CAD build for the part. Positions are in the model's coordinates, mm. Face numbers are marked on the shaded views. A direction names the side the tool comes from. Coordinates: 2 decimals unless noted, no trailing zeros. Write each loop counter-clockwise with the first axis right and the second up, starting at its lowest first coordinate (ties: lowest second). Pieces come first, ordered by that corner, then holes. Notation, with made-up numbers: M 28.25,63.25 L 77.25,63.25 A24 cw 77.25,73.25 Z; hole C -36.5,63.5 d1. An arc over 180 degrees is marked long. Put each result on its own line as item: value. Start each with the question number.
```python
from build123d import *

# Parameters (mm, degrees)
F0_W     = 139.7
F0_H     = 133.35
F1_DEPTH = 38.1
F2_T     = -1.5
F4_DEPTH = 1.5


# Not quite as in the source:
# - a pattern or mirror of a feature is missing from the dataset's text; its kind, count and spacing are read off the source's solid


with BuildPart() as f1:
    # F0 (on Top) → F1 (new body)
    with BuildSketch(Plane.XY):
        Rectangle(F0_W, F0_H)
    extrude(amount=F1_DEPTH)

    # F2
    f2_openings = [f1.faces().sort_by_distance(p)[0] for p in [
        (0, 0, 38.1),
    ]]
    offset(amount=F2_T, openings=f2_openings)

    # F3 (on face) → F4 (cut)
    with BuildSketch(Plane.XZ.offset(66.675)):
        with BuildLine():
            Line((19.05, 20.55), (-19.05, 20.55))
            ThreePointArc((-19.05, 20.55), (0, 1.5), (19.05, 20.55))
        make_face()
        with BuildLine():
            Line((-19.05, 38.1), (-19.05, 20.55))
            ThreePointArc((-19.05, 20.55), (-15.8753360228, 31.0797771184), (-7.4094534211, 38.1))
            Line((-7.4094534211, 38.1), (-19.05, 38.1))
        make_face()
        with BuildLine():
            ThreePointArc((-7.4094534211, 38.1), (-15.8753360228, 31.0797771184), (-19.05, 20.55))
            Line((-19.05, 20.55), (19.05, 20.55))
            ThreePointArc((19.05, 20.55), (15.8753360228, 31.0797771184), (7.4094534211, 38.1))
            Line((7.4094534211, 38.1), (-7.4094534211, 38.1))
        make_face()
        with BuildLine():
            ThreePointArc((7.4094534211, 38.1), (15.8753360228, 31.0797771184), (19.05, 20.55))
            Line((19.05, 20.55), (19.05, 38.1))
            Line((19.05, 38.1), (7.4094534211, 38.1))
        make_face()
        with BuildLine():
            ThreePointArc((7.4094534211, 38.1), (0, 39.6), (-7.4094534211, 38.1))
            Line((-7.4094534211, 38.1), (7.4094534211, 38.1))
        make_face()
    f4 = extrude(amount=-F4_DEPTH, mode=Mode.SUBTRACT)

    # F4_copies: F4 across plane
    add(f4.mirror(Plane.ZX), mode=Mode.SUBTRACT)


solid = f1.part
```
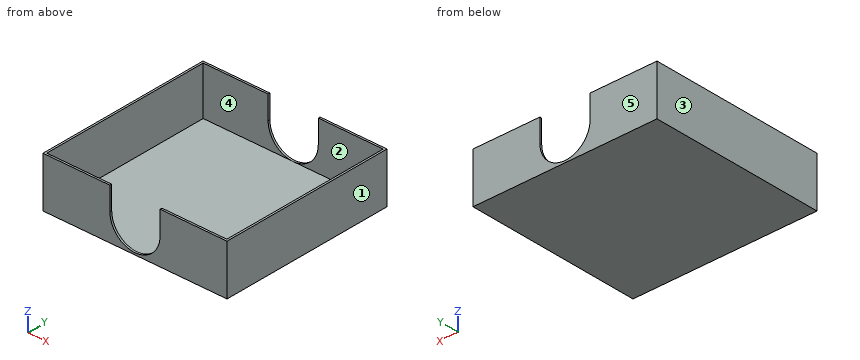
(1) Slice it at C-C, the plane x = -25.5. Write the cut outline in (y, z) (3 decimals), then the cut area to 3 significant figures.
(2) Two-plate mould, pull along Y, no slides. Class the marked faces 3, 4 and 5: +Y half, -Y half, draft (parallel to the pull), parting line (faces both ways), or undercut.
(3) Drill centre lines: line 1 (Y direction, x = 18.5, z = 13) (3 decimals); line 2 (X direction, y = 39, z = 18); line 3 (Z direction, x = 2.5, y = -55). Where is each one in solid material? Low to high. Write a range as [from, to].
(4) Slice it at B-B, the plane y = 47. Write the cut outline in (x, z).
(5) Which spindle directions (+Z, -Z, +X, -X, +Y, -Y) get a long thin tool onto all of the face, cutting with end or side? Do the marked faces 1 and 2. Say none if no direction does.
(6) Drop a flat-ended pin along its axis: pin 1 (12 mm diameter, centred on x = 31, y = -31, fed in from +Z). Give the stop position or say it passes through.
(7) Slice it at A-A, the plane z = 29.5. Write the cut outline in (x, y) (3 decimals).
(8) Slice it at D-D, the plane z = 15. Write the cut outline in (x, y) (3 decimals).
Result set:
1. outline: M -66.675,0 L 66.675,0 L 66.675,38.1 L 65.175,38.1 L 65.175,1.5 L -65.175,1.5 L -65.175,38.1 L -66.675,38.1 Z
1. area: 310 mm^2
2. face 3: draft
2. face 4: undercut
2. face 5: +Y half
3. line 1: y = [-66.675, -65.175], [65.175, 66.675]
3. line 2: x = [-69.85, -68.35], [68.35, 69.85]
3. line 3: z = [0, 1.5]
4. outline: M -69.85,0 L 69.85,0 L 69.85,38.1 L 68.35,38.1 L 68.35,1.5 L -68.35,1.5 L -68.35,38.1 L -69.85,38.1 Z
5. face 1: +Z, -Z, +X, +Y, -Y
5. face 2: +Z
6. pin 1: stops at z = 1.5
7. outline: M -69.85,-66.675 L -19.05,-66.675 L -19.05,-65.175 L -68.35,-65.175 L -68.35,65.175 L -19.05,65.175 L -19.05,66.675 L -69.85,66.675 Z; M 19.05,-66.675 L 69.85,-66.675 L 69.85,66.675 L 19.05,66.675 L 19.05,65.175 L 68.35,65.175 L 68.35,-65.175 L 19.05,-65.175 Z
8. outline: M -69.85,-66.675 L -18.224,-66.675 L -18.224,-65.175 L -68.35,-65.175 L -68.35,65.175 L -18.224,65.175 L -18.224,66.675 L -69.85,66.675 Z; M 18.224,-66.675 L 69.85,-66.675 L 69.85,66.675 L 18.224,66.675 L 18.224,65.175 L 68.35,65.175 L 68.35,-65.175 L 18.224,-65.175 Z
